Build history of the part. All positions in model axes, mm. A direction names the side the tool comes from. Give positions to 0.01 mm unless a question says otherwise; leave off trailing zeros. Order: outer loops, then holes, each group sorted by start corner. A loop starts at its lowest first (then second) coordinate and runs counter-clockwise, first axis right, second up. Notation, with made-up numbers: M 71,21.25 L 123,21.25 A15 ccw 123,49.25 Z; hole C -30.75,47 d9. An arc over 180 degrees is marked long. Answer as CSV lines item,"result".
from build123d import *

# Parameters (mm, degrees)
SKETCH_2_W               = 70
SKETCH_2_H               = 40
EXTRUDE_1_DEPTH          = 50
SKETCH_3_W               = 20
SKETCH_3_H               = 10
SKETCH_3_W_2             = 10
CUT_EXTRUDE_1_DEPTH      = 41
CUT_EXTRUDE_3_DEPTH      = 51
CUT_EXTRUDE_3_DEPTH_BACK = 1


with BuildPart() as part:
    # 草圖2 → 填料-伸長1 (new body)
    with BuildSketch(Plane(origin=(0, 0, 0), x_dir=(1, 0, 0), z_dir=(0, 1, 0))):
        Rectangle(SKETCH_2_W, SKETCH_2_H)
    extrude(amount=EXTRUDE_1_DEPTH)

    # 草圖3 → 除料-伸長1 (cut, through all)
    with BuildSketch(Plane.XY.offset(20)):
        with Locations((-25, 45)):
            Rectangle(SKETCH_3_W, SKETCH_3_H)
        with BuildLine():
            Line((5, 30), (35, 30))
            Line((35, 30), (35, 50))
            Line((35, 50), (-5, 50))
            Line((-5, 50), (-5, 40))
            ThreePointArc((-5, 40), (-2.071067812, 32.928932188), (5, 30))
        make_face()
        with BuildLine():
            Line((5, 10), (5, 0))
            Line((5, 0), (35, 0))
            Line((35, 0), (35, 20))
            Line((35, 20), (15, 20))
            ThreePointArc((15, 20), (7.928932188, 17.071067812), (5, 10))
        make_face()
        with Locations((-30, 5)):
            Rectangle(SKETCH_3_W_2, SKETCH_3_H)
    extrude(amount=-CUT_EXTRUDE_1_DEPTH, mode=Mode.SUBTRACT)

    # 草圖4 → 除料-伸長3 (cut, two sides)
    with BuildSketch(Plane(origin=(0, 0, 0), x_dir=(1, 0, 0), z_dir=(0, 1, 0))) as cut_extrude_3_sk:
        with BuildLine():
            Line((35, 20), (15, 20))
            ThreePointArc((15, 20), (29.142135624, 14.142135624), (35, 0))
            Line((35, 0), (35, 20))
        make_face()
        with BuildLine():
            Line((35, -20), (35, 0))
            ThreePointArc((35, 0), (29.142135624, -14.142135624), (15, -20))
            Line((15, -20), (35, -20))
        make_face()
    extrude(amount=CUT_EXTRUDE_3_DEPTH, mode=Mode.SUBTRACT)
    extrude(cut_extrude_3_sk.sketch, amount=-CUT_EXTRUDE_3_DEPTH_BACK, mode=Mode.SUBTRACT)


solid = part.part
Item 1: Band-saw the part on B-B (x = -23.5). Give the cut face in (y, z).
Geometry says:
outline,"M 0,-20 L 40,-20 L 40,20 L 0,20 Z"
Item 2: Drop flat-ended pins along their axis: pin 1 (22 mm diameter, centred on x = -24.5, z = 1, fed in from +Y); pin 2 (3 mm diameter, centred on x = 27.5, z = 5, fed in from +Y); pin 3 (5 mm diameter, centred on y = 43, z = 4, fed in from -X); pin 4 (6 mm diameter, centred on y = 34, z = 4, fed in from +X). Give the stop position or say it passes through.
Geometry says:
pin 1,"stops at y = 50"
pin 2,"stops at y = 30"
pin 3,"stops at x = -15"
pin 4,"stops at x = 0.64"
Item 3: Band-saw the part on A-A (z = 16). Give the cut face in (x, y), and give its area (3 significant figures).
Geometry says:
outline,"M -35,10 L -25,10 L -25,0 L 5,0 L 5,10 A10 cw 15,20 L 27,20 L 27,30 L 5,30 A10 cw -5,40 L -5,50 L -15,50 L -15,40 L -35,40 Z"
area,"1,760 mm2"
Item 4: 3-axis set-ups, long thin cutter, end or side, ignore diameter. For faces 1 (the flat face through (-30, 10, 0)), 2 (the flat face through (23, 20, 0)), 3 (the flat face through (-15, 45, 0)), 4 (the flat face through (16, 30, 0)): which of +Z, -Z, +X, -X, +Y, -Y reach the whole face in a straight line?
Geometry says:
face 1,"+Z, -Z, -X, -Y"
face 2,"+Z, -Z, +X, -Y"
face 3,"+Z, -Z, -X, +Y"
face 4,"+Z, -Z, +X, +Y"
Item 5: Band-saw the part on C-C (y = 16). Give the cut face in (x, z), and give its area (3 significant figures).
Geometry says:
outline,"M -35,-20 L 7,-20 L 7,20 L -35,20 Z"
area,"1,680 mm2"
Item 6: Probe line 1 along X through (y, z) = (5.5, -12.5); line 2 along Y through (x, z) = (-18, 14.5); line 3 along Y through (x, z) = (-28.5, -8.5). List the from-to ranges inside material, lowest first. Write a range as from..to.
Geometry says:
line 1,"x = -25..5"
line 2,"y = 0..40"
line 3,"y = 10..40"
Item 7: Band-saw the part on D-D (z = 12). Give the cut face in (x, y), and give its area (3 significant figures).
Geometry says:
outline,"M -35,10 L -25,10 L -25,0 L 5,0 L 5,10 A10 cw 15,20 L 31,20 L 31,30 L 5,30 A10 cw -5,40 L -5,50 L -15,50 L -15,40 L -35,40 Z"
area,"1,800 mm2"
